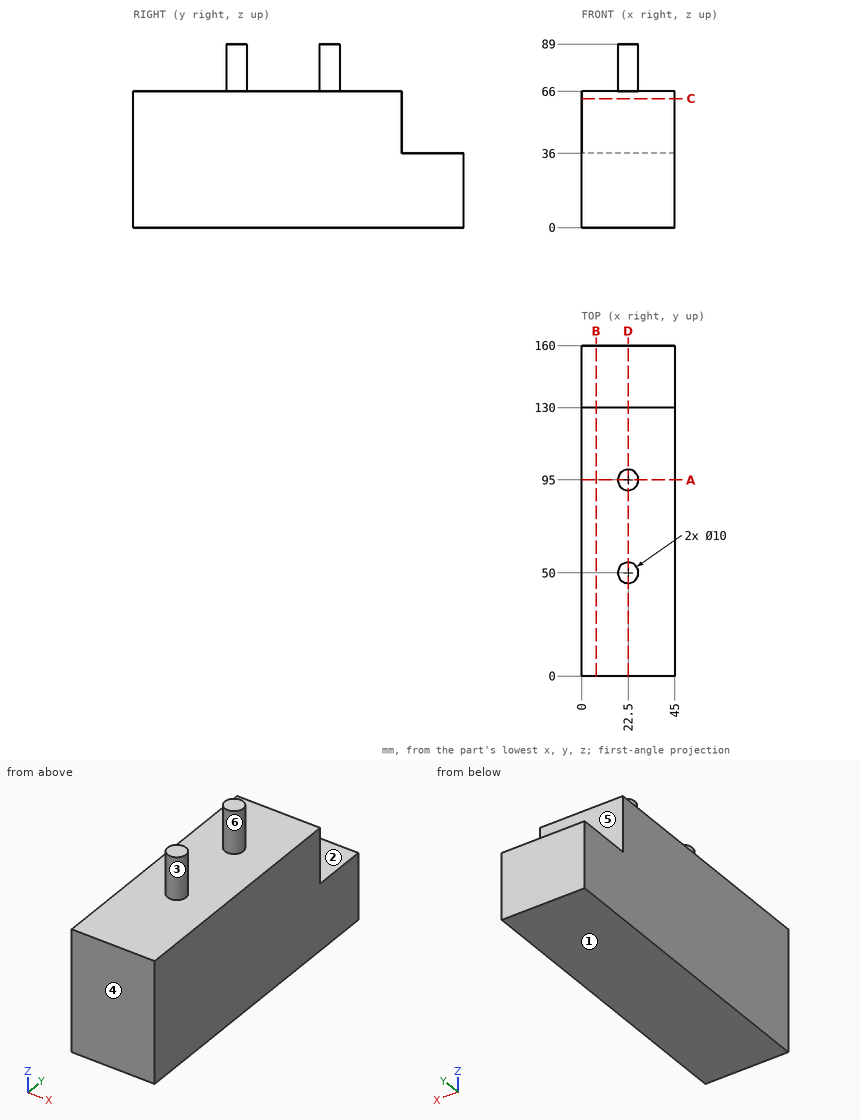
Job drawing, mm, ordinate dimensions from the low corner. One solid piece. A direction names the side the tool comes from. Give positions to 0.01 mm unless a question says otherwise; leave off trailing zeros. Loops run counter-clockwise (first coordinate to the right, second up) from the corner with the lowest first, then second, coordinate; pieces in that order, holes last. Notation, with made-up numbers: M -14,14 L 14,14 A26 ccw 14,52 Z; hole C 48.5,27.25 d10. An arc over 180 degrees is marked long. Answer in a Markdown table with one row per item. Add a question column.
Item 1: Probe probe 1 along Y at (x, z) = (22, 75); probe 2 along Z at (x, y) = (40, 89); probe 3 along Y at (x, z) = (8.5, 42). List the from-to ranges inside material, lowest first.
Item 2: Mould opens along Y. For the marked faces 4, 5 and 6 say: +Y half, -Y half, draft (parallel to the pull), parting line (faces both ways), or undercut.
Item 3: Band-saw the part on D-D on x = 22.5. Give the cut face in (y, z).
Item 4: Drop flat-ended pins along their axis: P1, Ø24, axis at x = 14.5, y = 150.5, coming from the +Z side; P2, Ø1, axis at x = 21, z = 72.5, coming from the +Y side; P3, Ø24, axis at x = 12.5, z = 49, coming from the +Y side. Give the stop position or say it passes through.
Item 5: Tool access for the marked faces 1, 2 and 3: list every direction of +Z, -Z, +X, -X, +Y, -Y with a clear straight run to the whole face (end or side of a thin tool).
Item 6: Band-saw the part on B-B on x = 7. Give the cut face in (y, z), then the cut area to 3 significant figures.
Item 7: Band-saw the part on C-C on z = 62.5. Give the cut face in (x, y).
Item 8: Band-saw the part on A-A on y = 95. Give the cut face in (x, z), then the cut area to 3 significant figures.
Reply:
| question | item | result |
|---|---|---|
| 1 | probe 1 | y = 45.03 to 54.97, 90.03 to 99.97 |
| 1 | probe 2 | z = 0 to 66 |
| 1 | probe 3 | y = 0 to 130 |
| 2 | face 4 | -Y half |
| 2 | face 5 | +Y half |
| 2 | face 6 | undercut |
| 3 | outline | M 0,0 L 160,0 L 160,36 L 130,36 L 130,66 L 100,66 L 100,89 L 90,89 L 90,66 L 55,66 L 55,89 L 45,89 L 45,66 L 0,66 Z |
| 4 | P1 | stops at z = 36 |
| 4 | P2 | stops at y = 99.9 |
| 4 | P3 | stops at y = 130 |
| 5 | face 1 | -Z, +X, -X, +Y, -Y |
| 5 | face 2 | +Z, +X, -X, +Y |
| 5 | face 3 | +Z |
| 6 | outline | M 0,0 L 160,0 L 160,36 L 130,36 L 130,66 L 0,66 Z |
| 6 | area | 9,660 mm^2 |
| 7 | outline | M 0,0 L 45,0 L 45,130 L 0,130 Z |
| 8 | outline | M 0,0 L 45,0 L 45,66 L 27.5,66 L 27.5,89 L 17.5,89 L 17.5,66 L 0,66 Z |
| 8 | area | 3,200 mm^2 |
